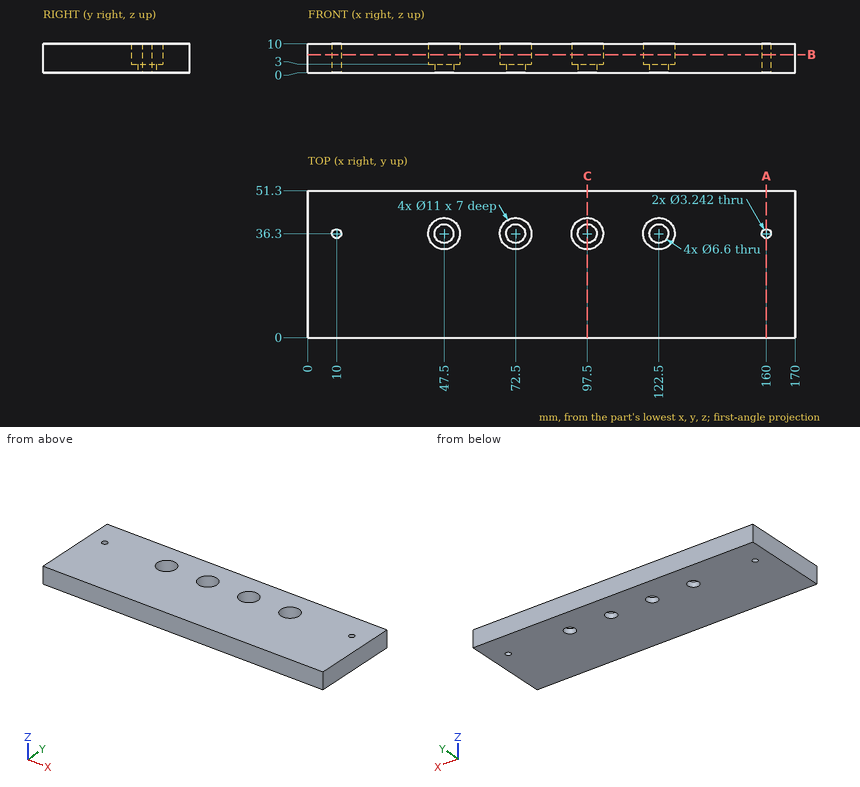
Verification items for this drawing (mm, ordinates from the low corner). Coordinates: 2 decimals unless noted, no trailing zeros. Order: outer loops, then holes, each group sorted by start corner. A loop starts at its lowest first (then second) coordinate and runs counter-clockwise, first axis right, second up. Notation, with made-up numbers: (30, -34.5) - (56, -34.5) arc R31 cw to (56, -1.5) - close; hole circle Ø3 at (-15, 40). An arc over 180 degrees is marked (long way). Answer as a JSON object with one key per item and string values. Group by question number.
Item 1: Sectioned sample at B-B, the plane z = 6.25. Record the cut outline in (x, y).
Item 2: Sectioned sample at C-C, the plane x = 97.5. Record the cut outline in (y, z).
Item 3: Scan lines: probe 1 along Y at (x, z) = (160, 7); probe 2 along Y at (x, z) = (97.5, 1.35); probe 3 along X at (y, z) = (39, 8). Record each from-to range of solid material in increasing order.
Item 4: Sectioned sample at A-A, the plane x = 160. Record the cut outline in (y, z), and give its area (3 significant figures).
Item 5: Depth check by flat-ended pin: pin 1 Ø5.5 at (x, y) = (120.5, 35.5) entering from +Z. Enter the tip coordinate at first touch or a pass-through.
Resolved:
{
 "1": {"outline": "(0, 0) - (170, 0) - (170, 51.3) - (0, 51.3) - close; hole circle Ø3.24 at (10, 36.3); hole circle Ø11 at (47.5, 36.3); hole circle Ø11 at (72.5, 36.3); hole circle Ø11 at (97.5, 36.3); hole circle Ø11 at (122.5, 36.3); hole circle Ø3.24 at (160, 36.3)"},
 "2": {"outline": "(0, 0) - (33, 0) - (33, 3) - (30.8, 3) - (30.8, 10) - (0, 10) - close; (39.6, 0) - (51.3, 0) - (51.3, 10) - (41.8, 10) - (41.8, 3) - (39.6, 3) - close"},
 "3": {"probe 1": "0 to 34.68, 37.92 to 51.3", "probe 2": "0 to 33, 39.6 to 51.3", "probe 3": "0 to 42.71, 52.29 to 67.71, 77.29 to 92.71, 102.29 to 117.71, 127.29 to 170"},
 "4": {"outline": "(0, 0) - (34.68, 0) - (34.68, 10) - (0, 10) - close; (37.92, 0) - (51.3, 0) - (51.3, 10) - (37.92, 10) - close", "area": "481 mm^2"},
 "5": {"pin 1": "z = 3"}
}
